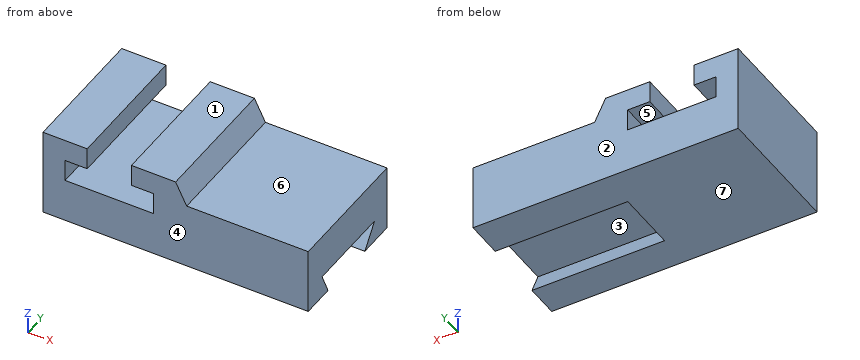
```python
from build123d import *

# Parameters (mm, degrees)
F1_DEPTH = 76.2
F3_DEPTH = 76.2


with BuildPart() as f1:
    # F0 (on Front) → F1 (new body)
    with BuildSketch(Plane.XZ):
        Polygon((0, 50.8), (0, 0), (152.4, 0), (152.4, 38.1), (82.55, 38.1), (76.2, 50.8), (50.8, 50.8), (50.8, 38.1), (63.5, 38.1), (63.5, 25.4), (12.7, 25.4), (12.7, 38.1), (25.4, 38.1), (25.4, 50.8), align=None)
    extrude(amount=-F1_DEPTH)

    # F2 (on face) → F3 (cut)
    with BuildSketch(Plane.YZ.offset(152.4)):
        Polygon((13.39724, 12.7), (19.161692, 0), (54.76566, 0), (64.19724, 12.7), align=None)
    extrude(amount=-F3_DEPTH, mode=Mode.SUBTRACT)


solid = f1.part
```
Part model, mm, in its own coordinate system. Face numbers are marked on the shaded views. A direction names the side the tool comes from. Coordinates: 2 decimals unless noted, no trailing zeros. Order: outer loops, then holes, each group sorted by start corner. A loop starts at its lowest first (then second) coordinate and runs counter-clockwise, first axis right, second up. Notation, with made-up numbers: (-33, 61) - (-15, 61) arc R13 ccw to (-15, 75) - close; hole circle Ø8 at (-6, -13). An arc over 180 degrees is marked (long way). Return JSON: item names as keys, results as strings. Group by question number.
Item 1: Pull direction Y, two halves, no side cores. Call the marked faces 1, 2, 3 and 4: pulls with the +Y half, pulls with the -Y half, needs draft (parallel to the pull), parting line crosses it, or undercut.
Item 2: Cut at D-D (y = 53). List the corners of the cut face in (x, z), plus the area to 3 significant figures.
Item 3: Pin check, flat tips, straight feed: pin 1 (12 mm diameter, centred on x = 106.5, y = 38, fed in from +Z); pin 2 (6.5 mm diameter, centred on y = 48, z = 5.5, fed in from +X). Stop position of each tip, or through.
Item 4: Cut at B-B (x = 19). List the corners of the cut face in (y, z), plus the area to 3 significant figures.
Item 5: Cut at A-A (z = 33). List the corners of the cut face in (x, y), plus the area to 3 significant figures.
Item 6: Drill centre lines: probe 1 along Z at (x, y) = (58, 50); probe 2 along X at (y, z) = (15, 26); probe 3 along X at (y, z) = (26, 41). Where is each one in solid material? Low to high. Write a range as from..to.
Item 7: Which spindle directions (+Z, -Z, +X, -X, +Y, -Y) get a long thin tool onto all of the face, cutting with end or side? Do the marked faces 5, 6 and 7. Say none if no direction does.
Item 8: Cut at C-C (x = 109). List the corners of the cut face in (y, z).
Check values:
{
 "1": {"face 1": "needs draft", "face 2": "pulls with the +Y half", "face 3": "undercut", "face 4": "pulls with the -Y half"},
 "2": {"outline": "(0, 0) - (76.2, 0) - (76.2, 12.7) - (152.4, 12.7) - (152.4, 38.1) - (82.55, 38.1) - (76.2, 50.8) - (50.8, 50.8) - (50.8, 38.1) - (63.5, 38.1) - (63.5, 25.4) - (12.7, 25.4) - (12.7, 38.1) - (25.4, 38.1) - (25.4, 50.8) - (0, 50.8) - close", "area": "4,880 mm2"},
 "3": {"pin 1": "stops at z = 38.1", "pin 2": "stops at x = 76.2"},
 "4": {"outline": "(0, 0) - (76.2, 0) - (76.2, 25.4) - (0, 25.4) - close; (0, 38.1) - (76.2, 38.1) - (76.2, 50.8) - (0, 50.8) - close", "area": "2,900 mm2"},
 "5": {"outline": "(0, 0) - (12.7, 0) - (12.7, 76.2) - (0, 76.2) - close; (63.5, 0) - (152.4, 0) - (152.4, 76.2) - (63.5, 76.2) - close", "area": "7,740 mm2"},
 "6": {"probe 1": "z = 0..25.4, 38.1..50.8", "probe 2": "x = 0..12.7, 63.5..152.4", "probe 3": "x = 0..25.4, 50.8..81.1"},
 "7": {"face 5": "+Y, -Y", "face 6": "+Z, +X, +Y, -Y", "face 7": "-Z, +X, -X, +Y, -Y"},
 "8": {"outline": "(0, 0) - (19.16, 0) - (13.4, 12.7) - (64.2, 12.7) - (54.77, 0) - (76.2, 0) - (76.2, 38.1) - (0, 38.1) - close"}
}
